Could you check a few things on this drawing? It's one solid part, dimensions in mm from its lowest x, y, z. Coordinates: 2 decimals unless noted, no trailing zeros. Order: outer loops, then holes, each group sorted by start corner. A loop starts at its lowest first (then second) coordinate and runs counter-clockwise, first axis right, second up. Notation, with made-up numbers: (-39, -10.5) - (-25, -10.5) arc R19 ccw to (-25, -5.5) - close; hole circle Ø4 at (86, -34.5). An arc over 180 degrees is marked (long way). Return JSON: item names as keys, results as strings. Group by question number.
1) If I drill on line 1 along X through (y, z) = (40, 97); line 2 along X through (y, z) = (37, 108); line 3 along Y through (x, z) = (84, 130.5), over which ranges is the centre line in solid material (lowest first)?
2) Imagine slicing it at D-D (z = 111). Write out the boundary of the cut face in (x, y).
3) If we mould it in two halves opening along X, with no side actions, what happens to the marked faces 1, 2 and 3? For each: pulls with the +X half, pulls with the -X half, needs draft (parallel to the pull), parting line crosses it, or undercut.
4) Imagine slicing it at C-C (x = 222.25). Write out the boundary of the cut face in (y, z), and give its area (3 significant figures).
5) Imagine slicing it at A-A (y = 43). Write out the boundary of the cut face in (x, z), and give its area (3 significant figures).
6) Imagine slicing it at B-B (z = 139.5). Write out the boundary of the cut face in (x, y), and give its area (3 significant figures).
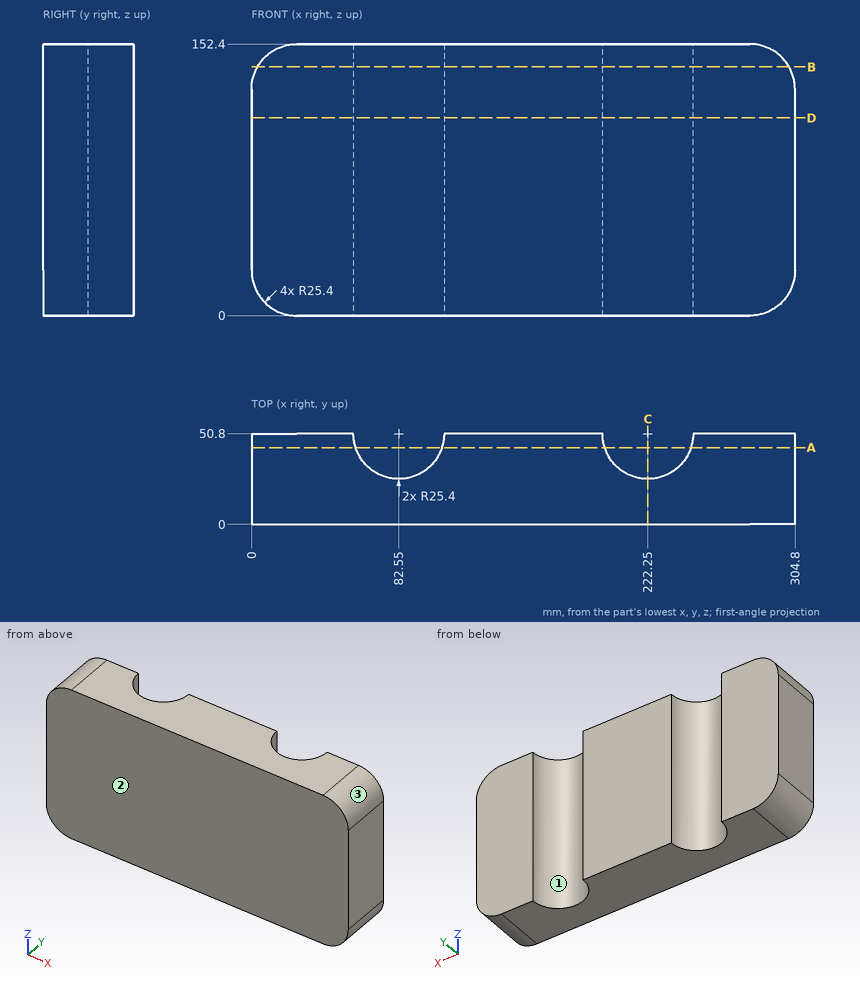
Calculated:
{
 "1": {"line 1": "0 to 59.56, 105.54 to 199.26, 245.24 to 304.8", "line 2": "0 to 61.23, 103.87 to 200.93, 243.57 to 304.8", "line 3": "0 to 25.44"},
 "2": {"outline": "(0, 0) - (304.8, 0) - (304.8, 50.8) - (247.65, 50.8) arc R25.4 cw to (196.85, 50.8) - (107.95, 50.8) arc R25.4 cw to (57.15, 50.8) - (0, 50.8) - close"},
 "3": {"face 1": "undercut", "face 2": "needs draft", "face 3": "pulls with the +X half"},
 "4": {"outline": "(0, 0) - (25.4, 0) - (25.4, 152.4) - (0, 152.4) - close", "area": "3,870 mm2"},
 "5": {"outline": "(0, 25.4) arc R25.4 ccw to (25.4, 0) - (58.38, 0) - (58.38, 152.4) - (25.4, 152.4) arc R25.4 ccw to (0, 127) - close; (106.72, 0) - (198.08, 0) - (198.08, 152.4) - (106.72, 152.4) - close; (246.42, 0) - (279.4, 0) arc R25.4 ccw to (304.8, 25.4) - (304.8, 127) arc R25.4 ccw to (279.4, 152.4) - (246.42, 152.4) - close", "area": "31,200 mm2"},
 "6": {"outline": "(3.29, 0) - (301.51, 0) - (301.51, 50.8) - (247.65, 50.8) arc R25.4 cw to (196.85, 50.8) - (107.95, 50.8) arc R25.4 cw to (57.15, 50.8) - (3.29, 50.8) - close", "area": "13,100 mm2"}
}
